Model file for the job. Use its own axes, mm. Face numbers are marked on the shaded views. A direction names the side the tool comes from. Round coordinates to 2 decimals unless told otherwise and drop trailing zeros. Order: outer loops, then holes, each group sorted by start corner. A loop starts at its lowest first (then second) coordinate and runs counter-clockwise, first axis right, second up. Notation, with made-up numbers: M 82.5,30.25 L 96.5,30.25 A20 ccw 96.5,43.25 Z; hole C 28,-21.5 d1. An arc over 180 degrees is marked long. Return JSON: item names as keys, results as strings. Group by question number.
Item 1: Slice it at C-C on x = 140. Write the cut outline in (y, z).
Item 2: Probe line 1 along Y through (x, z) = (3.5, 30); line 2 along Z through (x, y) = (150, -46); line 3 along X through (y, z) = (-46.4, 15.3). List the from-to ranges inside material, lowest first.
Item 3: Slice it at A-A on x = 88. Write the cut outline in (y, z).
Item 4: Pin check, flat tips, straight feed: pin 1 Ø3 at (x, y) = (16, 23) entering from +Z; pin 2 Ø0.9 at (x, y) = (68, -46.5) entering from -Z; pin 3 Ø3 at (x, z) = (38.5, 12.5) entering from +Y. Stop position of each tip, or through.
Item 5: Which spindle directions (+Z, -Z, +X, -X, +Y, -Y) get a long thin tool onto all of the face, cutting with end or side? Do the marked faces 1 and 2. Say none if no direction does.
Item 6: Pull direction Y, two halves, no side cores. Call the marked faces 3, 4 and 5: pulls with the +Y half, pulls with the -Y half, needs draft (parallel to the pull), parting line crosses it, or undercut.
Item 7: Slice it at B-B on z = 8. Write the cut outline in (x, y), then the cut area to 3 significant figures.
Item 8: Slice it at D-D on x = 56. Write the cut outline in (y, z).
from build123d import *

# Parameters (mm, degrees)
ESBO_O11_W                   = 30
ESBO_O11_H                   = 85.4
FLANGE_BASE1_DEPTH           = 3
FURO_DE_DI_METRO_3_2_3_2_1_D = 3.2
FURO_DE_DI_METRO_9_0_9_1_D   = 9
ARESTA_FLANGE1_DEPTH         = 30
ARESTA_FLANGE1_START         = 3
ARESTA_FLANGE1_PROFILE_R     = 1.6
ARESTA_FLANGE1_PROFILE_R_2   = 3
ARESTA_FLANGE1_FLAT_DEPTH    = 3
ARESTA_FLANGE2_DEPTH         = 30
ARESTA_FLANGE2_START         = 3
ARESTA_FLANGE2_PROFILE_R     = 1.6
ARESTA_FLANGE2_PROFILE_R_2   = 3
ARESTA_FLANGE2_FLAT_DEPTH    = 3
ESBO_O28_R                   = 1.6
CORTE_EXTRUS_O1_DEPTH        = 191.983899845


# Sheet-metal steps are written as plain solids
with BuildPart() as part:
    # Esboço11 → Flange-base1 (new body)
    with BuildSketch(Plane(origin=(0, 0, 0), x_dir=(-1, 0, 0), z_dir=(0, 0, -1))):
        with Locations((-4, 0)):
            Rectangle(ESBO_O11_W, ESBO_O11_H)
    extrude(amount=-FLANGE_BASE1_DEPTH)

    # Furo de diâmetro Ø3.2 (3.2)1 (through all)
    with Locations(Plane.XY.offset(3)):
        with Locations((0, 18), (0, 2)):
            Hole(FURO_DE_DI_METRO_3_2_3_2_1_D / 2)

    # Furo de diâmetro Ø9.0 (9)1 (through all)
    with Locations(Plane.XY.offset(3)):
        with Locations((0, 10)):
            Hole(FURO_DE_DI_METRO_9_0_9_1_D / 2)

    # Aresta-Flange1 bend section (across the edge) → Aresta-Flange1 (add)
    with BuildSketch(Plane(origin=(-11, -45, 3), x_dir=(0, 1, 0), z_dir=(1, 0, 0))):
        with BuildLine():
            Line((-3, 2.3), (0, 2.3))
            ThreePointArc((0, 2.3), (0.673654403, 0.673654403), (2.3, 0))
            Line((2.3, 0), (2.3, -3))
            ThreePointArc((2.3, -3), (-1.44766594, -1.44766594), (-3, 2.3))
        make_face()
    extrude(amount=ARESTA_FLANGE1_DEPTH)

    # Aresta-Flange1 profile (on flange) → Aresta-Flange1 flat (add)
    with BuildSketch(Plane(origin=(0, -45, 3), x_dir=(1, 0, 0), z_dir=(0, -1, 0)).offset(ARESTA_FLANGE1_START)):
        with BuildLine():
            Line((148.286348541, 43.289074758), (113.989303003, 49.156785916))
            ThreePointArc((113.989303003, 49.156785916), (113.149163903, 49.264132154), (112.302954462, 49.3))
            Line((112.302954462, 49.3), (72.176029381, 49.3))
            ThreePointArc((72.176029381, 49.3), (71.15753405, 49.247998153), (70.149631446, 49.092533452))
            Line((70.149631446, 49.092533452), (-3.026397935, 33.950001079))
            ThreePointArc((-3.026397935, 33.950001079), (-8.754481909, 30.471579625), (-11, 24.157467627))
            Line((-11, 24.157467627), (-11, 2.3))
            Line((-11, 2.3), (19, 2.3))
            ThreePointArc((19, 2.3), (20.464466094, 5.835533906), (24, 7.3))
            Line((24, 7.3), (146.6, 7.3))
            ThreePointArc((146.6, 7.3), (153.671067812, 10.228932188), (156.6, 17.3))
            Line((156.6, 17.3), (156.6, 33.432288841))
            ThreePointArc((156.6, 33.432288841), (154.244065849, 39.879633822), (148.286348541, 43.289074758))
        make_face()
        with Locations((150, 20.3)):
            Circle(ARESTA_FLANGE1_PROFILE_R, mode=Mode.SUBTRACT)
        with Locations((130, 20.3)):
            Circle(ARESTA_FLANGE1_PROFILE_R, mode=Mode.SUBTRACT)
        with Locations((116.90221, 23.3)):
            Circle(ARESTA_FLANGE1_PROFILE_R, mode=Mode.SUBTRACT)
        with Locations((67.40221, 23.3)):
            Circle(ARESTA_FLANGE1_PROFILE_R, mode=Mode.SUBTRACT)
        with Locations((140, 28.3)):
            Circle(ARESTA_FLANGE1_PROFILE_R_2, mode=Mode.SUBTRACT)
        with Locations((116.90221, 33.3)):
            Circle(ARESTA_FLANGE1_PROFILE_R, mode=Mode.SUBTRACT)
        with Locations((150, 36.3)):
            Circle(ARESTA_FLANGE1_PROFILE_R, mode=Mode.SUBTRACT)
        with Locations((130, 36.3)):
            Circle(ARESTA_FLANGE1_PROFILE_R, mode=Mode.SUBTRACT)
        with BuildLine():
            Line((115.15221, 30.3), (116.90221, 30.3))
            ThreePointArc((116.90221, 30.3), (118.90221, 28.3), (116.90221, 26.3))
            Line((116.90221, 26.3), (115.15221, 26.3))
            ThreePointArc((115.15221, 26.3), (113.737996438, 25.714213562), (113.15221, 24.3))
            Line((113.15221, 24.3), (113.15221, 17.3))
            Line((113.15221, 17.3), (71.15221, 17.3))
            Line((71.15221, 17.3), (71.15221, 24.3))
            ThreePointArc((71.15221, 24.3), (70.566423562, 25.714213562), (69.15221, 26.3))
            Line((69.15221, 26.3), (67.40221, 26.3))
            ThreePointArc((67.40221, 26.3), (65.40221, 28.3), (67.40221, 30.3))
            Line((67.40221, 30.3), (69.15221, 30.3))
            ThreePointArc((69.15221, 30.3), (70.566423562, 30.885786438), (71.15221, 32.3))
            Line((71.15221, 32.3), (71.15221, 39.3))
            Line((71.15221, 39.3), (113.15221, 39.3))
            Line((113.15221, 39.3), (113.15221, 32.3))
            ThreePointArc((113.15221, 32.3), (113.737996438, 30.885786438), (115.15221, 30.3))
        make_face(mode=Mode.SUBTRACT)
        with Locations((67.40221, 33.3)):
            Circle(ARESTA_FLANGE1_PROFILE_R, mode=Mode.SUBTRACT)
    extrude(amount=-ARESTA_FLANGE1_FLAT_DEPTH)

    # Aresta-Flange2 bend section (across the edge) → Aresta-Flange2 (add)
    with BuildSketch(Plane(origin=(19, 45, 3), x_dir=(0, -1, 0), z_dir=(-1, 0, 0))):
        with BuildLine():
            Line((-3, 2.3), (0, 2.3))
            ThreePointArc((0, 2.3), (0.673654403, 0.673654403), (2.3, 0))
            Line((2.3, 0), (2.3, -3))
            ThreePointArc((2.3, -3), (-1.44766594, -1.44766594), (-3, 2.3))
        make_face()
    extrude(amount=ARESTA_FLANGE2_DEPTH)

    # Aresta-Flange2 profile (on flange) → Aresta-Flange2 flat (add)
    with BuildSketch(Plane(origin=(0, 45, 3), x_dir=(-1, 0, 0), z_dir=(0, 1, 0)).offset(ARESTA_FLANGE2_START)):
        with BuildLine():
            ThreePointArc((-118.587276174, 38.294035384), (-121.912170898, 38.908863825), (-124.842101896, 40.596597007))
            ThreePointArc((-124.842101896, 40.596597007), (-127.832972518, 42.306539483), (-131.226645302, 42.9))
            Line((-131.226645302, 42.9), (-146.6, 42.9))
            ThreePointArc((-146.6, 42.9), (-153.671067812, 39.971067812), (-156.6, 32.9))
            Line((-156.6, 32.9), (-156.6, 23.656178366))
            ThreePointArc((-156.6, 23.656178366), (-153.716782168, 16.631122382), (-146.729717684, 13.657019735))
            Line((-146.729717684, 13.657019735), (-23.935141158, 12.064022895))
            ThreePointArc((-23.935141158, 12.064022895), (-20.441608916, 10.576971572), (-19, 7.06444358))
            Line((-19, 7.06444358), (-19, 2.3))
            Line((-19, 2.3), (11, 2.3))
            Line((11, 2.3), (11, 26.741804962))
            ThreePointArc((11, 26.741804962), (8.116782168, 33.766860946), (1.129717684, 36.740963592))
            Line((1.129717684, 36.740963592), (-118.587276174, 38.294035384))
        make_face()
        with Locations((-130, 20.3)):
            Circle(ARESTA_FLANGE2_PROFILE_R, mode=Mode.SUBTRACT)
        with Locations((-150, 20.3)):
            Circle(ARESTA_FLANGE2_PROFILE_R, mode=Mode.SUBTRACT)
        with Locations((-130, 36.3)):
            Circle(ARESTA_FLANGE2_PROFILE_R, mode=Mode.SUBTRACT)
        with Locations((-140, 28.3)):
            Circle(ARESTA_FLANGE2_PROFILE_R_2, mode=Mode.SUBTRACT)
        with Locations((-150, 36.3)):
            Circle(ARESTA_FLANGE2_PROFILE_R, mode=Mode.SUBTRACT)
    extrude(amount=-ARESTA_FLANGE2_FLAT_DEPTH)

    # Esboço28 → Corte-extrusão1 (cut, through all)
    with BuildSketch(Plane.XZ.offset(48)):
        with Locations(Location((-4, 15.3, 0), (0, 0, 270))):
            Circle(ESBO_O28_R)
        with Locations(Location((12, 15.3, 0), (0, 0, 270))):
            Circle(ESBO_O28_R)
    extrude(amount=-CORTE_EXTRUS_O1_DEPTH, mode=Mode.SUBTRACT)


solid = part.part
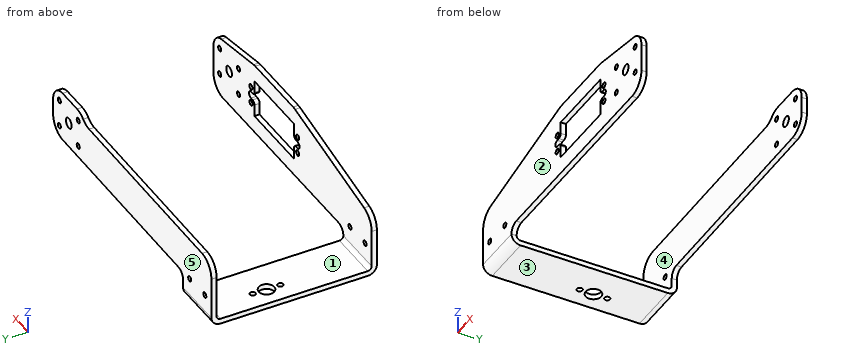
Output values:
{
 "1": {"outline": "M -48,10.3 L -45,10.3 L -45,28.3 L -48,28.3 Z; M -48,34.3 L -45,34.3 L -45,47.71 L -48,47.71 Z; M 45,16.57 L 48,16.57 L 48,28.3 L 45,28.3 Z; M 45,34.3 L 48,34.3 L 48,45.9 L 45,45.9 Z"},
 "2": {"line 1": "-48 to -45, 45 to 48", "line 2": "10.9 to 21.7, 24.9 to 37.7, 40.9 to 45.84", "line 3": "-11 to -5.6, -2.4 to 10.4, 13.6 to 155.26"},
 "3": {"outline": "M -48,10.3 L -45,10.3 L -45,20.3 L -48,20.3 Z; M -48,42.3 L -45,42.3 L -45,52.3 L -48,52.3 Z; M 45,15.9 L 48,15.9 L 48,40.9 L 45,40.9 Z"},
 "4": {"pin 1": "z = 3", "pin 2": "z = 10.3", "pin 3": "y = -45"},
 "5": {"face 1": "+Z, +X, -X", "face 2": "+Z, -Z, +X, -X, -Y"},
 "6": {"face 3": "needs draft", "face 4": "undercut", "face 5": "pulls with the +Y half"},
 "7": {"outline": "M -11,-48 L 19.79,-48 L 19.79,-45 L -11,-45 Z; M -11,45 L 19,45 L 19,48 L -11,48 Z", "area": "182 mm²"},
 "8": {"outline": "M -48,10.3 L -45,10.3 L -45,49.16 L -48,49.16 Z; M 45,15.48 L 48,15.48 L 48,40.48 L 45,40.48 Z"}
}
